Design review of the part built by this model. Coordinates are the model's own, in mm. Face numbers are marked on the shaded views. A direction names the side the tool comes from. Coordinates: 2 decimals unless noted, no trailing zeros. Loops run counter-clockwise (first coordinate to the right, second up) from the corner with the lowest first, then second, coordinate; pieces in that order, holes last. Notation, with made-up numbers: (28, 79) -> (60, 79) arc R18 ccw to (60, 93) -> close; hole circle Ø1 at (-18.5, 1). An arc over 180 degrees is marked (long way). Use one line per item in the form item = value. Start each with the question number.
1. The part is to be moulded in two halves that separate along Y. For the marked faces 5, 6 and 7, say which applies: released by +Y, released by -Y, zero draft, split by the parting line, or undercut.
2. Consider section C-C (z = -22.5). State the section outline as (x, y) points.
3. Wall thickness on line 1 (Z direction, x = -45, y = -41); line 2 (Y direction, x = 0, z = -15); line 3 (X direction, y = -47.5, z = 20): over which ranges is each line inside the solid? List them lowest first. Write a range as from..to.
4. For pin 1 (4 mm diameter, centred on y = -12.5, z = 4.5, fed in from +X); pin 2 (14 mm diameter, centred on x = -28.5, y = 15.5, fed in from +Z); pin 3 (11.5 mm diameter, centred on x = -45, z = 20, fed in from +Y); pin 4 (16 mm diameter, centred on x = 0, y = 32, fed in from -Z), all flat-tipped, find the tip position at first contact; note any pin that passes through.
5. Consider section B-B (x = 35). State the section outline as (y, z) points, then the cut area to 3 significant figures.
6. Consider section D-D (y = -34). State the section outline as (x, z) points, then the cut area to 3 significant figures.
7. Machinability: for the marked faces 1, 2, 3 and 4, which of the approach directions +Z, -Z, +X, -X, +Y, -Y give a long, thin tool a straight path to every point of the face, cutting with its end or side? Answer none if there is none.
8. Consider section A-A (z = 16.5). State the section outline as (x, y) points.
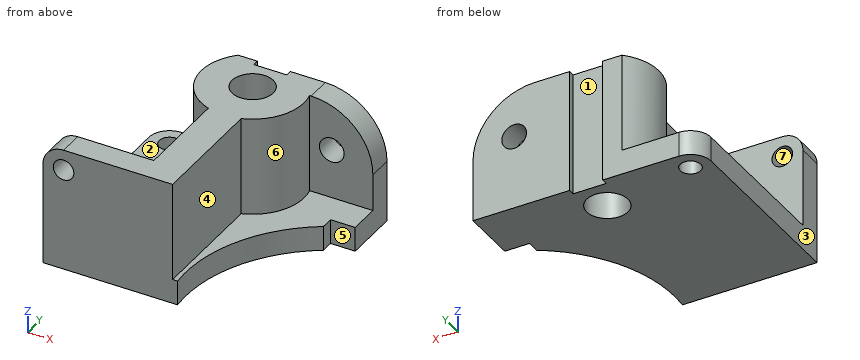
from build123d import *

# Parameters (mm, degrees)
SKETCH1_W           = 110
SKETCH1_H           = 100
BOSS_EXTRUDE1_DEPTH = 30
CUT_EXTRUDE1_DEPTH  = 48
SKETCH3_W           = 12
SKETCH3_H           = 6
CUT_EXTRUDE2_DEPTH  = 96.524865873
CUT_EXTRUDE5_DEPTH  = 48
CUT_EXTRUDE6_DEPTH  = 96.524865873
HOLE1_D             = 20
FILLET1_R           = 10
FILLET2_R           = 30
HOLE2_D             = 12
HOLE3_D             = 10
HOLE4_D             = 10
SKETCH15_W          = 16
SKETCH15_H          = 3
CUT_EXTRUDE7_DEPTH  = 96.524865873


with BuildPart() as part:
    # Sketch1 → Boss-Extrude1 (new, symmetric)
    with BuildSketch(Plane.XY):
        Rectangle(SKETCH1_W, SKETCH1_H)
    extrude(amount=BOSS_EXTRUDE1_DEPTH, both=True)

    # Sketch2 → Cut-Extrude1 (cut)
    with BuildSketch(Plane.XY.offset(30)):
        with BuildLine():
            Line((-8, 8.314561435), (-8, -38))
            Line((-8, -38), (-55, -38))
            Line((-55, -38), (-55, 50))
            Line((-55, 50), (-17.349351573, 50))
            ThreePointArc((-17.349351573, 50), (-24.393981909, 26.528834985), (-8, 8.314561435))
        make_face()
    extrude(amount=-CUT_EXTRUDE1_DEPTH, mode=Mode.SUBTRACT)

    # Sketch3 → Cut-Extrude2 (cut, through all)
    with BuildSketch(Plane.XY.offset(30)):
        with Locations((49, 20)):
            Rectangle(SKETCH3_W, SKETCH3_H)
    extrude(amount=-CUT_EXTRUDE2_DEPTH, mode=Mode.SUBTRACT)

    # Sketch4 → Cut-Extrude5 (cut)
    with BuildSketch(Plane.XY.offset(30)):
        with BuildLine():
            Line((8, -50), (10.411371468, -50))
            ThreePointArc((10.411371468, -50), (17.051338909, -11.804150412), (43, 17))
            Line((43, 17), (43, 23))
            Line((43, 23), (55, 23))
            Line((55, 23), (55, 38))
            Line((55, 38), (24.269322199, 38))
            ThreePointArc((24.269322199, 38), (21.92335751, 19.984743219), (8, 8.314561435))
            Line((8, 8.314561435), (8, -50))
        make_face()
    extrude(amount=-CUT_EXTRUDE5_DEPTH, mode=Mode.SUBTRACT)

    # Sketch6 → Cut-Extrude6 (cut, through all)
    with BuildSketch(Plane.XY.offset(30)):
        with BuildLine():
            Line((55, -50), (55, 17))
            Line((55, 17), (43, 17))
            ThreePointArc((43, 17), (17.051338909, -11.804150412), (10.411371468, -50))
            Line((10.411371468, -50), (55, -50))
        make_face()
    extrude(amount=-CUT_EXTRUDE6_DEPTH, mode=Mode.SUBTRACT)

    # Hole1 (through all)
    with Locations(Plane.XY.offset(30)):
        with Locations((0, 32)):
            Hole(HOLE1_D / 2)

    # Fillet1
    fillet1_edges = [part.edges().sort_by_distance(p)[0] for p in [
        (-55, -44, 30),
        (-55, 50, -24),
    ]]
    fillet(fillet1_edges, radius=FILLET1_R)

    # Fillet2
    fillet2_edges = [part.edges().sort_by_distance(p)[0] for p in [
        (55, 44, 30),
    ]]
    fillet(fillet2_edges, radius=FILLET2_R)

    # Hole2 (through all)
    with Locations(Plane(origin=(0, 50, 0), x_dir=(1, 0, 0), z_dir=(0, 1, 0))):
        with Locations((35, -6)):
            Hole(HOLE2_D / 2)

    # Hole3 (through all)
    with Locations(Plane(origin=(0, -38, 0), x_dir=(1, 0, 0), z_dir=(0, 1, 0))):
        with Locations((-45, -20)):
            Hole(HOLE3_D / 2)

    # Hole4 (through all)
    with Locations(Plane.XY.offset(-18)):
        with Locations((-45, 40)):
            Hole(HOLE4_D / 2)

    # Sketch15 → Cut-Extrude7 (cut, through all)
    with BuildSketch(Plane.XY.offset(30)):
        with Locations((0, 48.5)):
            Rectangle(SKETCH15_W, SKETCH15_H)
    extrude(amount=-CUT_EXTRUDE7_DEPTH, mode=Mode.SUBTRACT)


solid = part.part
Geometry check:
q1.face_5 = released by -Y
q1.face_6 = undercut
q1.face_7 = zero draft
q2.outline = (-55, -50) -> (10.41, -50) arc R70 cw to (43, 17) -> (43, 23) -> (55, 23) -> (55, 50) -> (8, 50) -> (8, 47) -> (-8, 47) -> (-8, 50) -> (-45, 50) arc R10 ccw to (-55, 40) -> close; hole circle Ø10 at (-45, 40); hole circle Ø20 at (0, 32)
q3.line_1 = -30..15, 25..30
q3.line_2 = -50..22, 42..47
q3.line_3 = -55..-50, -40..8
q4.pin_1 = 8
q4.pin_2 = -18
q4.pin_3 = -38
q4.pin_4 = through
q5.outline = (11.2, -30) -> (50, -30) -> (50, 0) -> (38, 0) -> (38, -18) -> (11.2, -18) -> close; (38, 12) -> (50, 12) -> (50, 28.28) -> (38, 28.28) -> close
q5.area = 877 mm²
q6.outline = (-55, -30) -> (10.51, -30) -> (10.51, -18) -> (8, -18) -> (8, 30) -> (-8, 30) -> (-8, -18) -> (-55, -18) -> close
q6.area = 1,550 mm²
q7.face_1 = +Z, -Z, +Y
q7.face_2 = +Z, -X
q7.face_3 = +Z, -Z, -X, +Y, -Y
q7.face_4 = +Z, +X, -Y
q8.outline = (-55, -50) -> (-48.57, -50) -> (-48.57, -38) -> (-55, -38) -> close; (-41.43, -50) -> (8, -50) -> (8, 8.31) arc R25 ccw to (24.27, 38) -> (50.05, 38) -> (50.05, 50) -> (8, 50) -> (8, 47) -> (-8, 47) -> (-8, 50) -> (-17.35, 50) arc R25 ccw to (-8, 8.31) -> (-8, -38) -> (-41.43, -38) -> close; hole circle Ø20 at (0, 32)
